Design review of the part built by this model. Coordinates are the model's own, in mm. Face numbers are marked on the shaded views. A direction names the side the tool comes from. Coordinates: 2 decimals unless noted, no trailing zeros. Write each loop counter-clockwise with the first axis right and the second up, starting at its lowest first coordinate (ties: lowest second). Pieces come first, ordered by that corner, then holes. Notation, with made-up numbers: (67, -8.75) - (92, -8.75) arc R19 ccw to (92, 19.25) - close; hole circle Ø3 at (3, 10). An arc over 180 degrees is marked (long way). Answer as a JSON object with one key per item and string values.
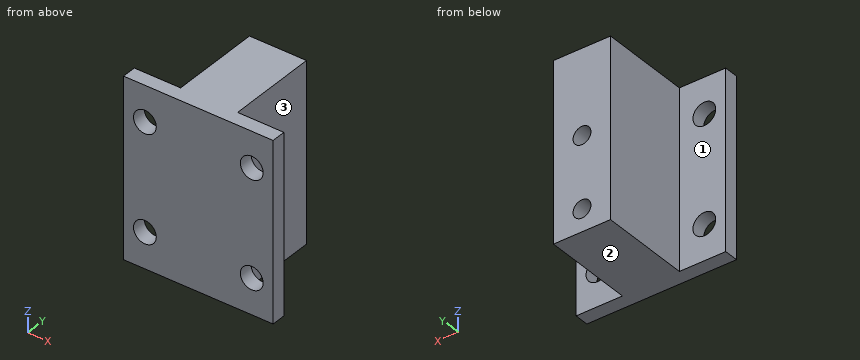
```python
from build123d import *

# Parameters (mm, degrees)
SKETCH1_W                 = 25
SKETCH1_H                 = 25
BOSS_EXTRUDE1_DEPTH       = 14.8
M3_CLEARANCE_HOLE1_D      = 3.2
M3X0_5_TAPPED_HOLE2_D     = 2.5
M3X0_5_TAPPED_HOLE2_DEPTH = 7.5
M3X0_5_TAPPED_HOLE2_TIP   = 0.751075774
SKETCH8_W                 = 8.5
SKETCH8_H                 = 25
CUT_EXTRUDE1_DEPTH        = 9.77
SKETCH9_W                 = 8.5
SKETCH9_H                 = 25
CUT_EXTRUDE2_DEPTH        = 9.77
SKETCH10_W                = 2
SKETCH10_H                = 25
CUT_EXTRUDE3_DEPTH        = 9.77
SKETCH11_W                = 2
SKETCH11_H                = 25
CUT_EXTRUDE4_DEPTH        = 9.77
SKETCH16_W                = 6.5
SKETCH16_H                = 25
CUT_EXTRUDE6_DEPTH        = 3.03
SKETCH17_W                = 6.5
SKETCH17_H                = 25
CUT_EXTRUDE7_DEPTH        = 3.03


with BuildPart() as part:
    # Sketch1 → Boss-Extrude1 (new body)
    with BuildSketch(Plane(origin=(0, 0, 0), x_dir=(1, 0, 0), z_dir=(0, 1, 0))):
        with Locations((12.5, -12.5)):
            Rectangle(SKETCH1_W, SKETCH1_H)
    extrude(amount=BOSS_EXTRUDE1_DEPTH)

    # M3 Clearance Hole1 (through all)
    with Locations(Plane(origin=(5, 14.8, 5), x_dir=(0, 0, 1), z_dir=(0, 1, 0))):
        with Locations((0, 0), (0, 15), (15, 15), (15, 0)):
            Hole(M3_CLEARANCE_HOLE1_D / 2)

    # M3x0.5 Tapped Hole2
    with Locations(Plane(origin=(12.5, 14.8, 3.124233191), x_dir=(0, 0, 1), z_dir=(0, 1, 0))):
        with Locations((0, 0), (10, 0)):
            Hole(M3X0_5_TAPPED_HOLE2_D / 2, depth=M3X0_5_TAPPED_HOLE2_DEPTH)
            with Locations((0, 0, -(M3X0_5_TAPPED_HOLE2_DEPTH + M3X0_5_TAPPED_HOLE2_TIP / 2))):  # 118° drill point
                Cone(0, M3X0_5_TAPPED_HOLE2_D / 2, M3X0_5_TAPPED_HOLE2_TIP, mode=Mode.SUBTRACT)

    # Sketch8 → Cut-Extrude1 (cut)
    with BuildSketch(Plane(origin=(0, 14.8, 0), x_dir=(1, 0, 0), z_dir=(0, 1, 0))):
        with Locations((4.25, -12.5)):
            Rectangle(SKETCH8_W, SKETCH8_H)
    extrude(amount=-CUT_EXTRUDE1_DEPTH, mode=Mode.SUBTRACT)

    # Sketch9 → Cut-Extrude2 (cut)
    with BuildSketch(Plane(origin=(0, 14.8, 0), x_dir=(1, 0, 0), z_dir=(0, 1, 0))):
        with Locations((20.75, -12.5)):
            Rectangle(SKETCH9_W, SKETCH9_H)
    extrude(amount=-CUT_EXTRUDE2_DEPTH, mode=Mode.SUBTRACT)

    # Sketch10 → Cut-Extrude3 (cut)
    with BuildSketch(Plane(origin=(0, 5.03, 0), x_dir=(1, 0, 0), z_dir=(0, 1, 0))):
        with Locations((1, -12.5)):
            Rectangle(SKETCH10_W, SKETCH10_H)
    extrude(amount=-CUT_EXTRUDE3_DEPTH, mode=Mode.SUBTRACT)

    # Sketch11 → Cut-Extrude4 (cut)
    with BuildSketch(Plane(origin=(0, 5.03, 0), x_dir=(1, 0, 0), z_dir=(0, 1, 0))):
        with Locations((24, -12.5)):
            Rectangle(SKETCH11_W, SKETCH11_H)
    extrude(amount=-CUT_EXTRUDE4_DEPTH, mode=Mode.SUBTRACT)

    # Sketch16 → Cut-Extrude6 (cut)
    with BuildSketch(Plane(origin=(0, 5.03, 0), x_dir=(1, 0, 0), z_dir=(0, 1, 0))):
        with Locations((5.25, -12.5)):
            Rectangle(SKETCH16_W, SKETCH16_H)
    extrude(amount=-CUT_EXTRUDE6_DEPTH, mode=Mode.SUBTRACT)

    # Sketch17 → Cut-Extrude7 (cut)
    with BuildSketch(Plane(origin=(0, 5.03, 0), x_dir=(1, 0, 0), z_dir=(0, 1, 0))):
        with Locations((19.75, -12.5)):
            Rectangle(SKETCH17_W, SKETCH17_H)
    extrude(amount=-CUT_EXTRUDE7_DEPTH, mode=Mode.SUBTRACT)


solid = part.part
```
(1) To check wall thickness, follow line 1 (Z direction, x = 12.5, y = 12); line 2 (X direction, y = 9, z = 23); line 3 (Y direction, x = 20.75, z = 10.25). State the ranges of each line that lie inside material, in increasing order. Write a range as from..to.
Solved:
{"line 1": "z = 0..1.87, 4.37..11.87, 14.37..25", "line 2": "x = 8.5..16.5", "line 3": "y = 0..2"}
(2) Take a section at C-C, the plane y = 9.75. Write out the cut boundary in (x, z), and give its area (3 significant figures).
Solved:
{"outline": "(8.5, 0) - (16.5, 0) - (16.5, 25) - (8.5, 25) - close; hole circle Ø2.5 at (12.5, 3.12); hole circle Ø2.5 at (12.5, 13.12)", "area": "190 mm^2"}
(3) Take a section at D-D, the plane z = 16. Write out the cut boundary in (x, y), and give its area (3 significant figures).
Solved:
{"outline": "(2, 0) - (23, 0) - (23, 2) - (16.5, 2) - (16.5, 14.8) - (8.5, 14.8) - (8.5, 2) - (2, 2) - close", "area": "144 mm^2"}
(4) Tool access review of the marked faces 1, 2 and 3: name each direction out of +Z, -Z, +X, -X, +Y, -Y from which nothing blocks a thin tool from reaching the whole face with its end or side.
Solved:
{"face 1": "+Z, -Z, -X, +Y", "face 2": "-Z, +X, -X, +Y, -Y", "face 3": "+Z, -Z, +X, +Y"}
(5) Take a section at A-A, the plane x = 20. Write out the cut boundary in (y, z), and give its area (3 significant figures).
Solved:
{"outline": "(0, 0) - (2, 0) - (2, 3.4) - (0, 3.4) - close; (0, 6.6) - (2, 6.6) - (2, 18.4) - (0, 18.4) - close; (0, 21.6) - (2, 21.6) - (2, 25) - (0, 25) - close", "area": "37.2 mm^2"}
(6) For pin 1 (4 mm diameter, centred on x = 20, z = 20, fed in from -Y); pin 2 (1 mm diameter, centred on y = 4.5, z = 6.5, fed in from +X); pin 3 (3 mm diameter, centred on x = 20, z = 5, fed in from -Y); pin 4 (3 mm diameter, centred on x = 18.5, z = 18, fed in from +Y), all flat-tipped, find the tip position at first contact; note any pin that passes through.
Solved:
{"pin 1": "stops at y = 0", "pin 2": "stops at x = 16.5", "pin 3": "passes through", "pin 4": "stops at y = 2"}
(7) Take a section at B-B, the plane z = 20. Write out the cut boundary in (x, y).
Solved:
{"outline": "(2, 0) - (3.4, 0) - (3.4, 2) - (2, 2) - close; (6.6, 0) - (18.4, 0) - (18.4, 2) - (16.5, 2) - (16.5, 14.8) - (8.5, 14.8) - (8.5, 2) - (6.6, 2) - close; (21.6, 0) - (23, 0) - (23, 2) - (21.6, 2) - close"}
